Geometry: final body of the model. Coordinates: model frame, mm. A direction names the side the tool comes from. Give positions to 0.01 mm unless a question says otherwise; leave off trailing zeros. Loops run counter-clockwise (first coordinate to the right, second up) from the corner with the lowest first, then second, coordinate; pieces in that order, holes last.
1. First-contact query: P1, Ø17.5, axis at y = -195.5, z = 537, coming from the -X side; P2, Ø11, axis at y = -200, z = 590.5, coming from the +X side. Flat tips, straight axial feed; report the tip coordinate or a pass-through.
2. Material intervals for line 1 along X through (y, z) = (-368, 810); line 2 along Y through (x, z) = (24, 766), sorted ascending.
3. Draft query along Y for faces 1 (the face through (-750, -15, 765)), 2 (the face through (726, 1100, 800)), 3 (the face through (10, 1023, 800)). Return one class per face: +Y half, -Y half, draft (parallel to the pull), parting line (faces both ways), or undercut.
4. Section A-A, the plane z = 466.5. Output: boundary loops of the cut face in (x, y), then the cut area to 3 significant figures.
5. Access query for faces 4 (the face through (-750, -15, 767)), 5 (the face through (-775, -15, 800)), 6 (the face through (-725, 1000, 800)), 7 (the face through (725, 1063, 800)), 8 (the face through (10, 975, 800)). Directions: +Z, -Z, +X, -X, +Y, -Y. A direction counts if a zero-diameter tool reaches every point of the face in a straight line with its end or side. Return the directions, or none.
6. Section B-B, the plane y = -757. Output: boundary loops of the cut face in (x, z).
7. Section C-C, the plane x = -319. Output: boundary loops of the cut face in (y, z).
from build123d import *

# Parameters (mm, degrees)
F0_W     = 46
F0_H     = 66
F1_DEPTH = 1100
F2_W     = 46
F2_H     = 66
F3_DEPTH = 725
F5_W     = 36
F5_H     = 36
F6_DEPTH = 350


with BuildPart() as f1:
    # F0 (on Front) → F1 (new body, symmetric)
    with BuildSketch(Plane.XZ):
        with BuildLine():
            ThreePointArc((775, 832.46), (774.256051, 834.256051), (772.46, 835))
            Line((772.46, 835), (727.54, 835))
            ThreePointArc((727.54, 835), (725.743949, 834.256051), (725, 832.46))
            Line((725, 832.46), (725, 767.54))
            ThreePointArc((725, 767.54), (725.743949, 765.743949), (727.54, 765))
            Line((727.54, 765), (772.46, 765))
            ThreePointArc((772.46, 765), (774.256051, 765.743949), (775, 767.54))
            Line((775, 767.54), (775, 832.46))
        make_face()
        with Locations((750, 800)):
            Rectangle(F0_W, F0_H, mode=Mode.SUBTRACT)
        with BuildLine():
            ThreePointArc((-727.54, 765), (-725.743949, 765.743949), (-725, 767.54))
            Line((-725, 767.54), (-725, 832.46))
            ThreePointArc((-725, 832.46), (-725.743949, 834.256051), (-727.54, 835))
            Line((-727.54, 835), (-772.46, 835))
            ThreePointArc((-772.46, 835), (-774.256051, 834.256051), (-775, 832.46))
            Line((-775, 832.46), (-775, 767.54))
            ThreePointArc((-775, 767.54), (-774.256051, 765.743949), (-772.46, 765))
            Line((-772.46, 765), (-727.54, 765))
        make_face()
        with Locations((-750, 800)):
            Rectangle(F0_W, F0_H, mode=Mode.SUBTRACT)
    extrude(amount=F1_DEPTH, both=True)

    # F2 (on Right) → F3 (join, symmetric)
    with BuildSketch(Plane.YZ):
        with BuildLine():
            ThreePointArc((1025, 832.46), (1024.256051, 834.256051), (1022.46, 835))
            Line((1022.46, 835), (977.54, 835))
            ThreePointArc((977.54, 835), (975.743949, 834.256051), (975, 832.46))
            Line((975, 832.46), (975, 767.54))
            ThreePointArc((975, 767.54), (975.743949, 765.743949), (977.54, 765))
            Line((977.54, 765), (1022.46, 765))
            ThreePointArc((1022.46, 765), (1024.256051, 765.743949), (1025, 767.54))
            Line((1025, 767.54), (1025, 832.46))
        make_face()
        with Locations((1000, 800)):
            Rectangle(F2_W, F2_H, mode=Mode.SUBTRACT)
    extrude(amount=F3_DEPTH, both=True)

    # F5 (on offset) → F6 (join)
    with BuildSketch(Plane.XY.offset(765)):
        with BuildLine():
            Line((767.46, -180), (732.54, -180))
            ThreePointArc((732.54, -180), (730.743949, -180.743949), (730, -182.54))
            Line((730, -182.54), (730, -217.46))
            ThreePointArc((730, -217.46), (730.743949, -219.256051), (732.54, -220))
            Line((732.54, -220), (767.46, -220))
            ThreePointArc((767.46, -220), (769.256051, -219.256051), (770, -217.46))
            Line((770, -217.46), (770, -182.54))
            ThreePointArc((770, -182.54), (769.256051, -180.743949), (767.46, -180))
        make_face()
        with Locations((750, -200)):
            Rectangle(F5_W, F5_H, mode=Mode.SUBTRACT)
        with BuildLine():
            ThreePointArc((-730, -182.54), (-730.743949, -180.743949), (-732.54, -180))
            Line((-732.54, -180), (-767.46, -180))
            ThreePointArc((-767.46, -180), (-769.256051, -180.743949), (-770, -182.54))
            Line((-770, -182.54), (-770, -217.46))
            ThreePointArc((-770, -217.46), (-769.256051, -219.256051), (-767.46, -220))
            Line((-767.46, -220), (-732.54, -220))
            ThreePointArc((-732.54, -220), (-730.743949, -219.256051), (-730, -217.46))
            Line((-730, -217.46), (-730, -182.54))
        make_face()
        with Locations((-750, -200)):
            Rectangle(F5_W, F5_H, mode=Mode.SUBTRACT)
    extrude(amount=-F6_DEPTH)


solid = f1.part
Answers below:
1. P1: stops at x = -770
1. P2: stops at x = 770
2. line 1: x = -775 to -773, -727 to -725, 725 to 727, 773 to 775
2. line 2: y = 975.52 to 1024.48
3. face 1: draft
3. face 2: +Y half
3. face 3: undercut
4. outline: (-770, -217.46) arc R2.54 ccw to (-767.46, -220) - (-732.54, -220) arc R2.54 ccw to (-730, -217.46) - (-730, -182.54) arc R2.54 ccw to (-732.54, -180) - (-767.46, -180) arc R2.54 ccw to (-770, -182.54) - close; (730, -217.46) arc R2.54 ccw to (732.54, -220) - (767.46, -220) arc R2.54 ccw to (770, -217.46) - (770, -182.54) arc R2.54 ccw to (767.46, -180) - (732.54, -180) arc R2.54 ccw to (730, -182.54) - close; hole (-768, -218) - (-732, -218) - (-732, -182) - (-768, -182) - close; hole (732, -218) - (768, -218) - (768, -182) - (732, -182) - close
4. area: 597 mm2
5. face 4: +Y, -Y
5. face 5: +Z, -Z, -X, +Y, -Y
5. face 6: none
5. face 7: +Z, -Z, +Y
5. face 8: +Z, -Z, -Y
6. outline: (-775, 767.54) arc R2.54 ccw to (-772.46, 765) - (-727.54, 765) arc R2.54 ccw to (-725, 767.54) - (-725, 832.46) arc R2.54 ccw to (-727.54, 835) - (-772.46, 835) arc R2.54 ccw to (-775, 832.46) - close; (725, 767.54) arc R2.54 ccw to (727.54, 765) - (772.46, 765) arc R2.54 ccw to (775, 767.54) - (775, 832.46) arc R2.54 ccw to (772.46, 835) - (727.54, 835) arc R2.54 ccw to (725, 832.46) - close; hole (-773, 767) - (-727, 767) - (-727, 833) - (-773, 833) - close; hole (727, 767) - (773, 767) - (773, 833) - (727, 833) - close
7. outline: (975, 767.54) arc R2.54 ccw to (977.54, 765) - (1022.46, 765) arc R2.54 ccw to (1025, 767.54) - (1025, 832.46) arc R2.54 ccw to (1022.46, 835) - (977.54, 835) arc R2.54 ccw to (975, 832.46) - close; hole (977, 767) - (1023, 767) - (1023, 833) - (977, 833) - close
